Autodesk Inventor part; units mm, degrees
ref_plane "YZ Plane" through (0, 0, 0) normal (1, 0, 0) x (0, 1, 0)
ref_plane "XZ Plane" through (0, 0, 0) normal (0, 1, 0) x (-1, 0, 0)
ref_plane "XY Plane" through (0, 0, 0) normal (0, 0, 1) x (1, 0, 0)
sketch "Sketch1" plane through (0, 0, 0) normal (1, 0, 0) x (0, 1, 0)
  line L0 (0, 0) -> (0, -139.8524)
  line L1 (0, 0) -> (-16.51, 0)
  line L2 (-16.51, 0) -> (-16.51, -31.75)
  line L3 (-16.51, -31.75) -> (-26.67, -31.75)
  line L4 (-26.67, -31.75) -> (-26.67, 10.16)
  line L5 (-26.67, 10.16) -> (10.16, 10.16)
  line L6 (10.16, 10.16) -> (10.16, -139.8524)
  line L7 (10.16, -139.8524) -> (0, -139.8524)
  dimension "d1" = 10.16
  dimension "d2" = 10.16
  dimension "d3" = 16.51
  dimension "d4" = 31.75
  dimension "d5" = 10.16
  dimension "d17" = 150.0124
extrude "Extrusion1" add sketch "Sketch1" along normal blind 10.16
sketch "Sketch2" plane through (0, 10.16, 10.16) normal (0, 1, 0) x (1, 0, 0)
  line L0 (2.54, 23.3934) -> (7.62, 23.3934)
  line L1 (7.62, 23.3934) -> (7.62, 42.4434)
  line L2 (7.62, 42.4434) -> (2.54, 42.4434)
  line L3 (2.54, 42.4434) -> (2.54, 23.3934)
  line L4 (0, 0) -> (10.16, 0)
  line L5 (0, 150.0124) -> (0, 0)
  line L6 (10.16, 150.0124) -> (10.16, 0)
  line L7 (2.54, 65.8368) -> (7.62, 65.8368)
  line L8 (7.62, 65.8368) -> (7.62, 84.8868)
  line L9 (7.62, 84.8868) -> (2.54, 84.8868)
  line L10 (2.54, 84.8868) -> (2.54, 65.8368)
  line L11 (2.54, 108.2802) -> (7.62, 108.2802)
  line L12 (7.62, 108.2802) -> (7.62, 127.3302)
  line L13 (7.62, 127.3302) -> (2.54, 127.3302)
  line L14 (2.54, 127.3302) -> (2.54, 108.2802)
  line L15 (0, 150.0124) -> (10.16, 150.0124)
  point P0 (0, 10.16)
  dimension "d8" = 23.3934
  dimension "d9" = 19.05
  dimension "d10" = 5.08
  dimension "d11" = 2.54
  dimension "d12" = 2.54
  dimension "d13" = 19.05
  dimension "d14" = 23.3934
  dimension "d15" = 19.05
  dimension "d16" = 23.3934
  dimension "d18" = 22.6822
  dimension "d19" = 5.08
  dimension "d20" = 5.08
  dimension "d21" = 2.54
  dimension "d22" = 2.54
  dimension "d23" = 2.54
  dimension "d24" = 2.54
extrude "Extrusion2" cut sketch "Sketch2" against normal blind 10.16 contours L3 L2 L1 L0 | L10 L9 L8 L7 | L14 L13 L12 L11
sketch "Sketch3" plane through (10.16, 0, 0) normal (1, 0, 0) x (0, 0, -1)
  line L0 (17.145, -24.13) -> (4.445, -24.13)
  line L1 (4.445, -24.13) -> (4.445, -19.05)
  line L2 (4.445, -19.05) -> (17.145, -19.05)
  line L3 (17.145, -19.05) -> (17.145, -24.13)
  line L4 (31.75, -16.51) -> (0, -16.51)
  line L5 (-10.16, -26.67) -> (31.75, -26.67)
  line L6 (-10.16, 10.16) -> (-10.16, -26.67)
  line L7 (31.75, -26.67) -> (31.75, -16.51)
  line L8 (-4.8133, 7.62) -> (7.8867, 7.62)
  line L9 (7.8867, 7.62) -> (7.8867, 2.54)
  line L10 (7.8867, 2.54) -> (-4.8133, 2.54)
  line L11 (-4.8133, 2.54) -> (-4.8133, 7.62)
  line L12 (139.8524, 10.16) -> (-10.16, 10.16)
  line L13 (0, 0) -> (139.8524, 0)
  line L14 (134.8613, 2.54) -> (122.1613, 2.54)
  line L15 (122.1613, 2.54) -> (122.1613, 7.62)
  line L16 (122.1613, 7.62) -> (134.8613, 7.62)
  line L17 (134.8613, 7.62) -> (134.8613, 2.54)
  line L18 (139.8524, 0) -> (139.8524, 10.16)
  line L19 (80.0735, 7.62) -> (92.7735, 7.62)
  line L20 (92.7735, 7.62) -> (92.7735, 2.54)
  line L21 (92.7735, 2.54) -> (80.0735, 2.54)
  line L22 (80.0735, 2.54) -> (80.0735, 7.62)
  line L23 (37.6301, 7.62) -> (50.3301, 7.62)
  line L24 (50.3301, 7.62) -> (50.3301, 2.54)
  line L25 (50.3301, 2.54) -> (37.6301, 2.54)
  line L26 (37.6301, 2.54) -> (37.6301, 7.62)
  point P0 (13.2334, 10.16)
  point P1 (117.1702, 10.16)
  point P2 (55.6768, 10.16)
  point P3 (32.2834, 10.16)
  point P4 (74.7268, 10.16)
  point P5 (98.1202, 10.16)
  dimension "d27" = 12.7
  dimension "d28" = 2.54
  dimension "d29" = 5.08
  dimension "d30" = 2.54
  dimension "d31" = 14.605
  dimension "d32" = 14.605
  dimension "d33" = 5.3467
  dimension "d34" = 12.7
  dimension "d35" = 5.3467
  dimension "d36" = 5.08
  dimension "d37" = 2.54
  dimension "d38" = 2.54
  dimension "d39" = 5.08
  dimension "d40" = 4.9911
  dimension "d41" = 12.7
  dimension "d42" = 4.9911
  dimension "d43" = 2.54
  dimension "d44" = 2.54
  dimension "d45" = 12.7
  dimension "d46" = 5.3467
  dimension "d47" = 5.3467
  dimension "d48" = 12.7
  dimension "d49" = 5.3467
  dimension "d50" = 5.3467
extrude "Extrusion3" cut sketch "Sketch3" against normal through all
equation "\"d2\" = d1"
equation "\"d11\" = d12"
equation "\"d13\" = d9"
equation "\"d14\" = d8"
equation "\"d15\" = d13"
equation "\"d16\" = d14"
equation "\"d28\" = d30"
equation "\"d31\" = d32"
equation "\"d37\" = d38"
equation "\"d43\" = d44"
properties part number "spool holder" material "PLA"
Work out the finished part from the listing and answer in its coordinate system (mm). A direction names the side the tool comes from. Give positions to 0.01 mm unless a question says otherwise; leave off trailing zeros. Write each loop counter-clockwise with the first axis right and the second up, starting at its lowest first coordinate (ties: lowest second). Pieces come first, ordered by that corner, then holes. Notation, with made-up numbers: (30, 77.5) - (50, 77.5) arc R12 cw to (50, 83.5) - close; hole circle Ø5 at (64, 4.5). An arc over 180 degrees is marked (long way). Use one line per item in the form item = value.
1. For faces 1 (the face through (5, -22, -31.75)), 2 (the face through (5, 5, -80.074)), 3 (the face through (7.62, 5, -65)), 4 (the face through (5, 5, -13.233)), 5 (the face through (5, -8, 0)), determine the directions among +Z, -Z, +X, -X, +Y, -Y from which every point of the face is accessible in a straight line to the end or side of a thin tool.
Filled in:
face_1 = -Z, +X, -X, -Y
face_2 = +X, -X
face_3 = +Y, -Y
face_4 = +Y
face_5 = -Z, +X, -X
2. A cutting plane is placed at C-C (y = -2). Write down the section's boundary in (x, z).
Filled in:
outline = (0, 0) - (10.16, 0) - (10.16, 10.16) - (0, 10.16) - close
3. A cutting plane is placed at B-B (x = 5.25). State how many separate pieces and enclosed holes the cut face has, and give its area (3 significant figures).
Filled in:
separate_pieces = 4
enclosed_holes = 5
area = 1,210 mm^2
4. A cutting plane is placed at A-A (z = -129). Write down the section's boundary in (x, y), and give its area (3 significant figures).
Filled in:
outline = (0, 0) - (10.16, 0) - (10.16, 2.54) - (0, 2.54) - close; (0, 7.62) - (10.16, 7.62) - (10.16, 10.16) - (0, 10.16) - close
area = 51.6 mm^2
5. Each of these flat-tipped pins is pushed along its axis until it touches: pin 1 Ø1 at (x, z) = (4.5, -65.5) entering from +Y; pin 2 Ø5 at (x, z) = (7, -39.5) entering from -Y; pin 3 Ø1.5 at (x, y) = (4.5, -21.5) entering from -Z. Where does it stop, or does it pass through?
Filled in:
pin_1 = through
pin_2 = 0
pin_3 = -31.75
6. Determine the mould class of faces 6 (the face through (7.62, 5, -23)), 7 (the face through (5, 5, 4.813)), 8 (the face through (8, 10.16, -64)) for opening direction Y: released by +Y, released by -Y, zero draft, split by the parting line, or undercut.
Filled in:
face_6 = zero draft
face_7 = undercut
face_8 = released by +Y
7. Consider L1, parallel to Z at x = 8, y = 7; L2, parallel to Y at x = 9.25, z = -5; L3, parallel to Y at x = 1.75, z = -8. Determine where each line is inside the solid, lowest interval first.
Filled in:
L1 = -139.85 to -134.86, -122.16 to -92.77, -80.07 to -50.33, -37.63 to -7.89, 4.81 to 10.16
L2 = -26.67 to -24.13, -19.05 to -16.51, 0 to 2.54, 7.62 to 10.16
L3 = -26.67 to -24.13, -19.05 to -16.51, 0 to 10.16
